Study the drawing (mm; zero at the part's minimum x, y, z) and answer. Round coordinates to 2 decimals unless told otherwise and drop trailing zeros. Order: outer loops, then holes, each group sorted by start corner. A loop starts at its lowest first (then second) coordinate and runs counter-clockwise, first axis right, second up. Notation, with made-up numbers: M 46,55 L 74,55 A28 cw 74,94 Z; hole C -12.75,36 d1. An arc over 180 degrees is marked long. Put each result on its own line as item: value. Start each with the question number.
1. The part is cut by section B-B (x = 1.45). Give the vertices of the cut face in (y, z).
2. The part is cut by section C-C (y = 11). Give the vertices of the cut face in (x, z).
3. The part is cut by section D-D (x = 3). Give the vertices of the cut face in (y, z), then the cut area to 3 significant figures.
4. Consider line 1 (Z direction, x = 3.1, y = 2.5); line 2 (Y direction, x = 1.2, z = 5.25); line 3 (X direction, y = 22, z = 2.45). Determine where each line is inside the solid, lowest interval first.
5. The mould has two halves that part along X. Classify the marked faces 1, 2 and 3: +X half, -X half, draft (parallel to the pull), parting line (faces both ways), or undercut.
6. Each of these flat-tipped pins is pushed along its axis until it touches: pin 1 Ø1 at (y, z) = (14, 1.5) entering from +X; pin 2 Ø1 at (x, z) = (2.5, 2) entering from +Y; pin 3 Ø2 at (x, y) = (1.5, 10.5) entering from -Z. Where does it stop, or does it pass through?
7. The part is cut by section A-A (z = 3). Give the vertices of the cut face in (x, y), then the cut area to 3 significant figures.
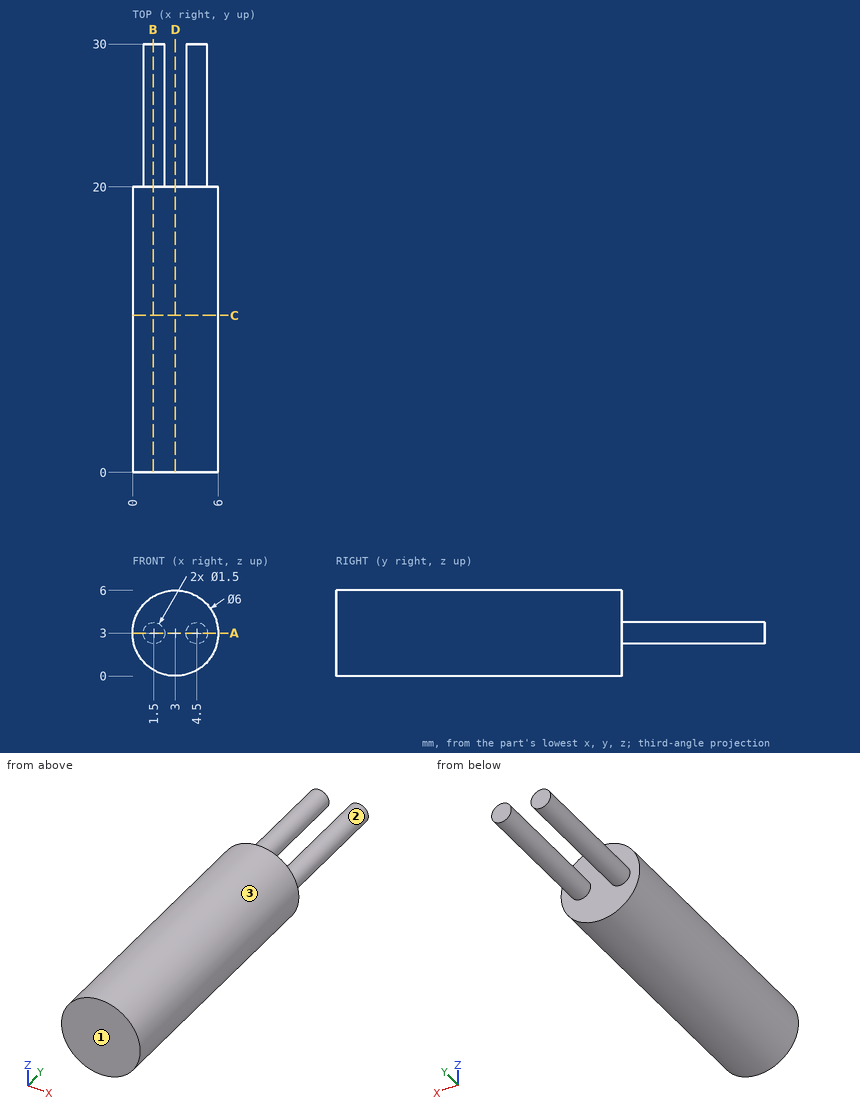
Resolved:
1. outline: M 0,0.43 L 20,0.43 L 20,2.25 L 30,2.25 L 30,3.75 L 20,3.75 L 20,5.57 L 0,5.57 Z
2. outline: C 3,3 d6
3. outline: M 0,0 L 20,0 L 20,6 L 0,6 Z
3. area: 120 mm2
4. line 1: 0 to 6
4. line 2: 0 to 20
4. line 3: 0.99 to 2.01, 3.99 to 5.01
5. face 1: draft
5. face 2: undercut
5. face 3: parting line
6. pin 1: x = 5.83
6. pin 2: y = 20
6. pin 3: z = 0.04
7. outline: M 0,0 L 6,0 L 6,20 L 5.25,20 L 5.25,30 L 3.75,30 L 3.75,20 L 2.25,20 L 2.25,30 L 0.75,30 L 0.75,20 L 0,20 Z
7. area: 150 mm2
